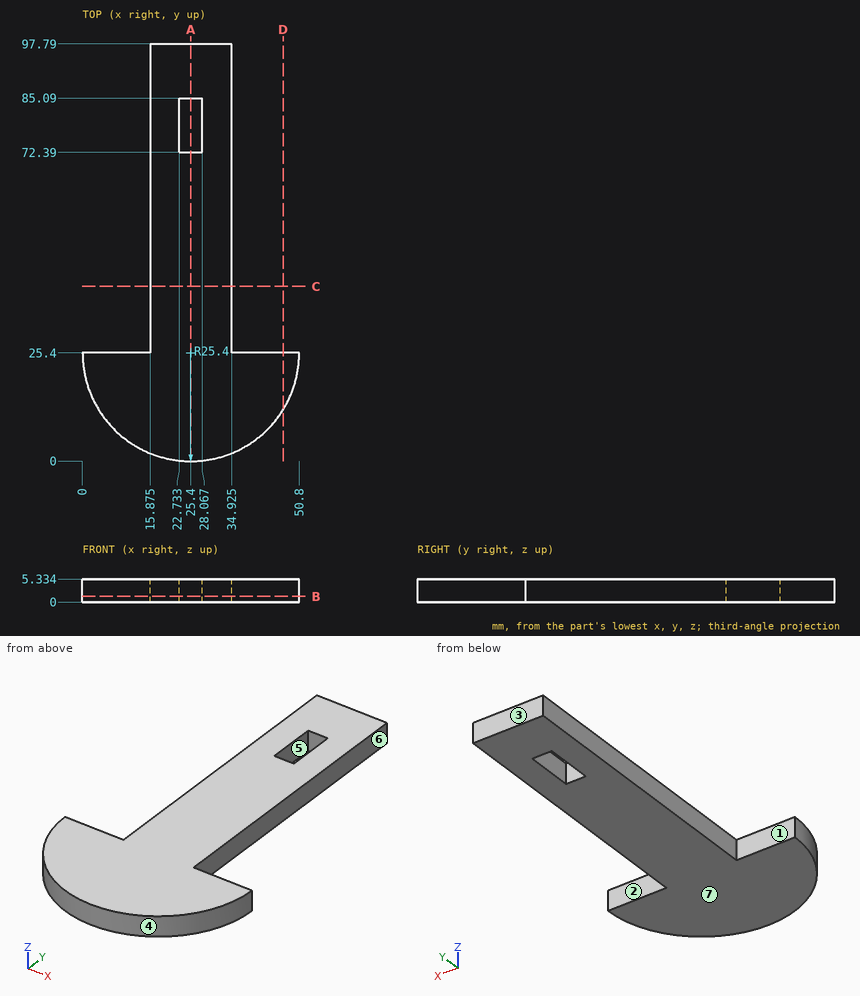
Check sheet for the drawn part. Datum: minimum x, y, z corner. Units: mm. A direction names the side the tool comes from. Round coordinates to 2 decimals unless told otherwise and drop trailing zeros. Order: outer loops, then holes, each group sorted by start corner. A loop starts at its lowest first (then second) coordinate and runs counter-clockwise, first axis right, second up. Notation, with made-up numbers: M 33.5,81.25 L 52.5,81.25 A5 ccw 52.5,87.25 Z; hole C 88,74.25 d7. An arc over 180 degrees is marked long. Write each question's results on one line, items separated by ' | '. Start each with the question number.
1. Cross-section at A-A on x = 25.4. Record the boundary of the cut face in (y, z), plus the area to 3 significant figures.
2. Cross-section at D-D on x = 47. Record the boundary of the cut face in (y, z).
3. Go/stop test with flat-tipped pins: P1, Ø1, axis at y = 66.5, z = 3.5, coming from the -X side (3 decimals); P2, Ø1.5, axis at x = 43, z = 1, coming from the +Y side; P3, Ø1.6, axis at y = 76.5, z = 3.5, coming from the +X side (3 decimals); P4, Ø6, axis at x = 38, y = 26.5, coming from the -Z side. Record where each tip stops, or that it passes through.
4. Set-up check for the marked faces 1, 2 and 3: record each of +Z, -Z, +X, -X, +Y, -Y from which the full face is reachable in a straight line by a thin tool's end or side.
5. Cross-section at C-C on y = 41. Record the boundary of the cut face in (x, z) (3 decimals), plus the area to 3 significant figures.
6. Material ranges on L1, parallel to X at y = 79, z = 0.75 (3 decimals); L2, parallel to Y at x = 25, z = 0.3; L3, parallel to X at y = 39.5, z = 3.2 (3 decimals), recorded low to high. Write a range as from..to.
7. Draft check along X on the marked faces 4, 5, 6 and 7. Enter one of: pulls with the +X half, pulls with the -X half, needs draft (parallel to the pull), parting line crosses it, or undercut.
8. Cross-section at B-B on z = 1.3. Record the boundary of the cut face in (x, y) (3 decimals).
Resolved:
1) outline: M 0,0 L 72.39,0 L 72.39,5.33 L 0,5.33 Z; M 85.09,0 L 97.79,0 L 97.79,5.33 L 85.09,5.33 Z | area: 454 mm2
2) outline: M 12.04,0 L 25.4,0 L 25.4,5.33 L 12.04,5.33 Z
3) P1: x = 15.875 | P2: y = 25.4 | P3: x = 34.925 | P4: z = 0
4) face 1: +Z, -Z, -X, +Y | face 2: +Z, -Z, +X, +Y | face 3: +Z, -Z, +X, -X, +Y
5) outline: M 15.875,0 L 34.925,0 L 34.925,5.334 L 15.875,5.334 Z | area: 102 mm2
6) L1: 15.875..22.733, 28.067..34.925 | L2: 0..72.39, 85.09..97.79 | L3: 15.875..34.925
7) face 4: parting line crosses it | face 5: undercut | face 6: pulls with the +X half | face 7: needs draft
8) outline: M 0,25.4 A25.4 ccw 50.8,25.4 L 34.925,25.4 L 34.925,97.79 L 15.875,97.79 L 15.875,25.4 Z; hole M 22.733,72.39 L 28.067,72.39 L 28.067,85.09 L 22.733,85.09 Z
